```python
from build123d import *

# Parameters (mm, degrees)
DODANIE_WYCI_GNI_CIE1_DEPTH = 6
SFAZOWANIE1_SIZE            = 3.5
ZAOKR_GLENIE1_R             = 1
SZKIC2_W                    = 11
SZKIC2_H                    = 5.5
WYTNIJ_WYCI_GNI_CIE1_DEPTH  = 5
SZKIC3_W                    = 9
SZKIC3_H                    = 6.5
WYTNIJ_WYCI_GNI_CIE2_DEPTH  = 4.5
SFAZOWANIE2_SIZE            = 0.5
SZKIC4_R                    = 5
DODANIE_WYCI_GNI_CIE2_DEPTH = 6
SZKIC5_W                    = 4
SZKIC5_H                    = 6
DODANIE_WYCI_GNI_CIE3_DEPTH = 4.5
SFAZOWANIE3_SIZE            = 3
SFAZOWANIE4_SIZE            = 1
ZAOKR_GLENIE2_R             = 2
SZKIC6_W                    = 43.68114346
SZKIC6_H                    = 110.382920914
WYTNIJ_WYCI_GNI_CIE3_DEPTH  = 0.5


with BuildPart() as part:
    # Szkic1 → Dodanie-wyciągnięcie1 (new body)
    with BuildSketch(Plane.XY):
        with BuildLine():
            ThreePointArc((15.75, 33.5), (0, 49.25), (-15.75, 33.5))
            Line((-15.75, 33.5), (15.75, 33.5))
        make_face()
        with BuildLine():
            Line((15.75, 33.5), (-15.75, 33.5))
            ThreePointArc((-15.75, 33.5), (0, 17.75), (15.75, 33.5))
        make_face()
        with BuildLine():
            ThreePointArc((15.75, 33.5), (0, 17.75), (-15.75, 33.5))
            Line((-15.75, 33.5), (-15.75, -33.5))
            Line((-15.75, -33.5), (15.75, -33.5))
            Line((15.75, -33.5), (15.75, 33.5))
        make_face()
    extrude(amount=-DODANIE_WYCI_GNI_CIE1_DEPTH)

    # Sfazowanie1
    # the kernel refuses this chamfer: 3.5 mm, written as the material it takes off along each edge
    with BuildSketch(Plane(origin=(15.75, -42.500890458, 0), x_dir=(-0.9996219169112968, 0, 0.02749587661058637), z_dir=(0, 1, 0)), Plane(origin=(-15.75, 33.5, 0), x_dir=(0.9996219169112968, 0, 0.02749587661058637), z_dir=(0, -1, 0)), Plane(origin=(-15.75, 33.5, -6), x_dir=(-0.02749587661058661, 0, 0.9996219169112968), z_dir=(0, -1, 0))) as sfazowanie1_piece_1:
        Polygon((SFAZOWANIE1_SIZE * 0.999621916911, -SFAZOWANIE1_SIZE * 0.0274958766106), (-SFAZOWANIE1_SIZE * 0.0274958766106, -SFAZOWANIE1_SIZE * 0.999621916911), (0, 0), align=None)
    extrude(amount=76.000890458, mode=Mode.SUBTRACT)
    with BuildSketch(Plane(origin=(15.75, -42.500890458, -6), x_dir=(-0.9996219169112968, 0, -0.027495876610586358), z_dir=(0, 1, 0))) as sfazowanie1_piece_2:
        Polygon((SFAZOWANIE1_SIZE * 0.999621916911, SFAZOWANIE1_SIZE * 0.0274958766106), (-SFAZOWANIE1_SIZE * 0.0274958766106, SFAZOWANIE1_SIZE * 0.999621916911), (0, 0), align=None)
    extrude(amount=76.000890458, mode=Mode.SUBTRACT)
    with BuildSketch(Plane(origin=(0, 33.5, 0), x_dir=(-1, 0, 0), z_dir=(0, -1, 0))) as sfazowanie1_piece_3:
        Polygon((15.75, SFAZOWANIE1_SIZE), (15.75 - SFAZOWANIE1_SIZE, 0), (15.75, 0), align=None)
    revolve(axis=Axis((0, 33.5, 0), (0, 0, -1)), revolution_arc=180, mode=Mode.SUBTRACT)
    with BuildSketch(Plane(origin=(0, 33.5, -6), x_dir=(1, 0, 0), z_dir=(0, -1, 0))) as sfazowanie1_piece_4:
        Polygon((15.75, SFAZOWANIE1_SIZE), (15.75 - SFAZOWANIE1_SIZE, 0), (15.75, 0), align=None)
    revolve(axis=Axis((0, 33.5, -6), (0, 0, 1)), revolution_arc=180, mode=Mode.SUBTRACT)

    # Zaokrąglenie1
    zaokr_glenie1_edges = [part.edges().sort_by_distance(p)[0] for p in [
        (-15.25, 0, -3),
        (0, 48.75, -3),
        (15.25, 0, -3),
    ]]
    fillet(zaokr_glenie1_edges, radius=ZAOKR_GLENIE1_R)

    # Szkic2 → Wytnij-wyciągnięcie1 (cut)
    with BuildSketch(Plane.XY):
        with Locations((5, 12.25)):
            Rectangle(SZKIC2_W, SZKIC2_H)
    extrude(amount=-WYTNIJ_WYCI_GNI_CIE1_DEPTH, mode=Mode.SUBTRACT)

    # Szkic3 → Wytnij-wyciągnięcie2 (cut)
    with BuildSketch(Plane(origin=(0, 0, -6), x_dir=(-1, 0, 0), z_dir=(0, 0, -1))):
        with Locations((6, -1.988867336)):
            Rectangle(SZKIC3_W, SZKIC3_H)
        with Locations((6, -27.988867336)):
            Rectangle(SZKIC3_W, SZKIC3_H)
    extrude(amount=-WYTNIJ_WYCI_GNI_CIE2_DEPTH, mode=Mode.SUBTRACT)

    # Sfazowanie2
    sfazowanie2_edges = [part.edges().sort_by_distance(p)[0] for p in [
        (-6, -24.738867336, -6),
    ]]
    chamfer(sfazowanie2_edges, length=SFAZOWANIE2_SIZE)

    # Szkic4 → Dodanie-wyciągnięcie2 (add)
    with BuildSketch(Plane.XY):
        with BuildLine():
            Line((9, -33.5), (-8.974684649, -33.5))
            Line((-8.974684649, -33.5), (-8.974684649, -43.705386779))
            ThreePointArc((-8.974684649, -43.705386779), (0.337519003, -52.024492564), (9, -43.030823629))
            Line((9, -43.030823629), (9, -33.5))
        make_face()
        with Locations((0, -43.030823629)):
            Circle(SZKIC4_R, mode=Mode.SUBTRACT)
    extrude(amount=-DODANIE_WYCI_GNI_CIE2_DEPTH)

    # Szkic5 → Dodanie-wyciągnięcie3 (add)
    with BuildSketch(Plane(origin=(0, 0, -6), x_dir=(-1, 0, 0), z_dir=(0, 0, -1))):
        with Locations((-2.5, 12)):
            Rectangle(SZKIC5_W, SZKIC5_H)
    extrude(amount=DODANIE_WYCI_GNI_CIE3_DEPTH)

    # Sfazowanie3
    sfazowanie3_edges = [part.edges().sort_by_distance(p)[0] for p in [
        (5, 15, 0),
    ]]
    chamfer(sfazowanie3_edges, length=SFAZOWANIE3_SIZE)

    # Sfazowanie4
    sfazowanie4_edges = [part.edges().sort_by_distance(p)[0] for p in [
        (5, 9.5, 0),
    ]]
    chamfer(sfazowanie4_edges, length=SFAZOWANIE4_SIZE)

    # Zaokrąglenie2
    zaokr_glenie2_edges = [part.edges().sort_by_distance(p)[0] for p in [
        (5, 9.5, -1),
    ]]
    fillet(zaokr_glenie2_edges, radius=ZAOKR_GLENIE2_R)

    # Szkic6 → Wytnij-wyciągnięcie3 (cut)
    with BuildSketch(Plane.XY):
        Rectangle(SZKIC6_W, SZKIC6_H)
    extrude(amount=-WYTNIJ_WYCI_GNI_CIE3_DEPTH, mode=Mode.SUBTRACT)


solid = part.part
```
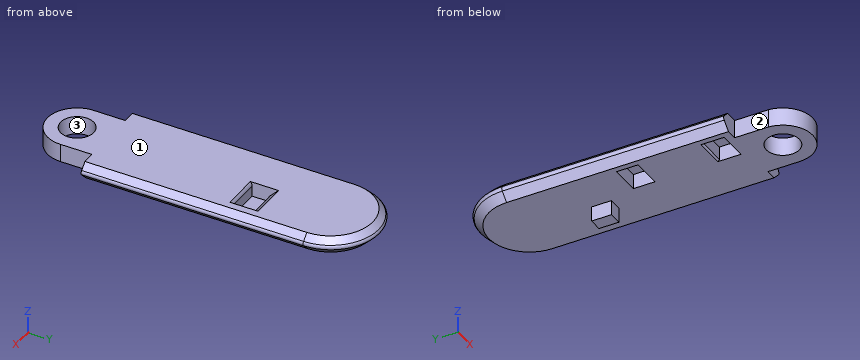
Build history of the part. All positions in model axes, mm. Face numbers are marked on the shaded views. Round coordinates to 2 decimals unless told otherwise and drop trailing zeros. Loops run counter-clockwise (first coordinate to the right, second up) from the corner with the lowest first, then second, coordinate; pieces in that order, holes last. Notation, with made-up numbers: M -39.75,-15.5 L 0.25,-15.5 A10 ccw 0.25,-6.5 Z; hole C 81.25,25 d7. An arc over 180 degrees is marked long. Answer as CSV lines item,"result".
1. Cut at B-B on y = 22.5. Write the cut outline in (x, z), then the cut area to 3 significant figures.
Resolved:
outline,"M -14.54,-3.71 L -12.25,-6 L 12.25,-6 L 14.54,-3.71 A1 ccw 14.54,-2.29 L 12.75,-0.5 L -12.75,-0.5 L -14.54,-2.29 A1 ccw Z"
area,"152 mm²"
2. Cut at A-A on y = -39.5. Write the cut outline in (x, z).
Resolved:
outline,"M -8.97,-6 L -3.54,-6 L -3.54,-0.5 L -8.97,-0.5 Z; M 3.54,-6 L 9,-6 L 9,-0.5 L 3.54,-0.5 Z"
3. Flat gauge pins, fed straight in: P1, Ø2, axis at x = 3.5, z = -4.5, coming from the -Y side; P2, Ø3, axis at y = -38.5, z = -3, coming from the -X side; P3, Ø4.5, axis at x = -12.5, z = -3.5, coming from the -Y side. Where does each tip first touch, or does it go through?
Resolved:
P1,"stops at y = -51.68"
P2,"stops at x = -8.97"
P3,"stops at y = -33.5"
4. Two-plate mould, pull along X, no slides. Class the marked faces 1, 2 and 3: released by +X, released by -X, zero draft, split by the parting line, or undercut.
Resolved:
face 1,"zero draft"
face 2,"released by -X"
face 3,"undercut"
5. Cut at C-C on z = -9.5. Write the cut outline in (x, y).
Resolved:
outline,"M 0.5,9 L 4.5,9 L 4.5,15 L 0.5,15 Z"
6. Wall check: probe 1 along Y at (x, z) = (0, -3.7); probe 2 along Y at (x, z) = (-3.5, -4.5); probe 3 along Y at (x, z) = (0, -3.35). Give the ranges that are in metal, low to high. Write a range as [from, to].
Resolved:
probe 1,"y = [-52.03, -48.03], [-38.03, 9.5], [15, 48.05]"
probe 2,"y = [-51.32, -46.6], [-39.46, -31.24], [-24.74, -5.24], [1.26, 46.8]"
probe 3,"y = [-52.03, -48.03], [-38.03, 9.5], [15, 48.27]"
